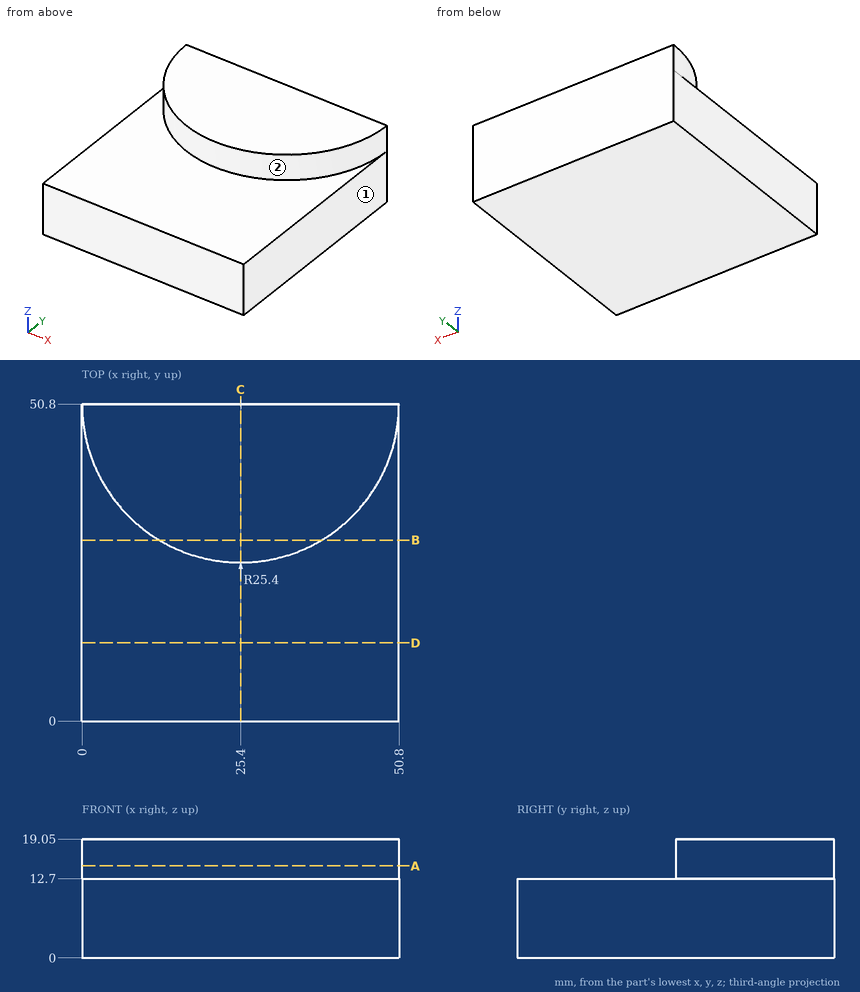
Geometry: see drawing. Coordinates: mm, zero at the bounding-box minimum. A direction names the side the tool comes from. Give positions to 0.01 mm unless a question says otherwise; leave off trailing zeros. Order: outer loops, then holes, each group sorted by start corner. A loop starts at its lowest first (then second) coordinate and runs counter-clockwise, first axis right, second up.
1. Pin query (flat end, axial travel): pin 1 Ø5 at (x, y) = (43.5, 16.5) entering from +Z. Return the tip coordinate at first contact, or that it passes through.
Computed:
pin 1: stops at z = 12.7
2. Line query: probe 1 along Z at (x, y) = (24.5, 14); probe 2 along Y at (x, z) = (38.5, 16.75); probe 3 along Y at (x, z) = (32, 16.75). Output: solid intervals per line, ascending.
Computed:
probe 1: z = 0 to 12.7
probe 2: y = 29.04 to 50.8
probe 3: y = 26.27 to 50.8
3. Set-up query: the marked faces 1 and 2. Return all of +Z, -Z, +X, -X, +Y, -Y with unobstructed straight access to the full face (end or side cutting, diameter ignored); none if empty.
Computed:
face 1: +Z, -Z, +X, +Y, -Y
face 2: +Z, -Y
4. Cut plane C-C (x = 25.4). Return loops of the section in (y, z), and give its area (3 significant figures).
Computed:
outline: (0, 0) - (50.8, 0) - (50.8, 19.05) - (25.4, 19.05) - (25.4, 12.7) - (0, 12.7) - close
area: 806 mm2
5. Cut plane D-D (y = 12.5). Return loops of the section in (x, z), and give its area (3 significant figures).
Computed:
outline: (0, 0) - (50.8, 0) - (50.8, 12.7) - (0, 12.7) - close
area: 645 mm2
6. Cut plane A-A (z = 14.75). Return loops of the section in (x, y), and give its area (3 significant figures).
Computed:
outline: (0, 50.8) arc R25.4 ccw to (50.8, 50.8) - close
area: 1,010 mm2
7. Cut plane B-B (y = 29). Return loops of the section in (x, z).
Computed:
outline: (0, 0) - (50.8, 0) - (50.8, 12.7) - (38.44, 12.7) - (38.44, 19.05) - (12.36, 19.05) - (12.36, 12.7) - (0, 12.7) - close
